Check sheet for the modelled part. Datum: model origin and axes. Units: mm. Face numbers are marked on the shaded views. A direction names the side the tool comes from. Round coordinates to 2 decimals unless told otherwise and drop trailing zeros. Loops run counter-clockwise (first coordinate to the right, second up) from the corner with the lowest first, then second, coordinate; pieces in that order, holes last. Notation, with made-up numbers: (62, 61.25) - (76, 61.25) arc R19 cw to (76, 96.25) - close; hole circle Ø3 at (88, 75). An arc over 180 degrees is marked (long way). Return JSON: item names as keys, results as strings.
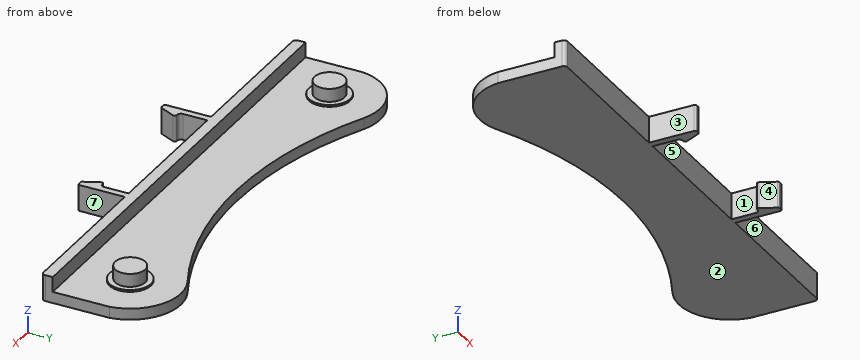
from build123d import *

# Parameters (mm, degrees)
F0_R     = 5.500353
F1_DEPTH = 3
F0_R_2   = 4.000323
F2_DEPTH = 3.5
F3_DEPTH = 7
F4_R     = 1
F5_R     = 0.5


with BuildPart() as f1:
    # F0 (on Top) → F1 (new body)
    with BuildSketch(Plane.XY):
        with BuildLine():
            ThreePointArc((0.003197, 9.6562), (-22.731522, 12.261138), (-44.2788, 19.966198))
            ThreePointArc((-44.2788, 19.966198), (-56.566858, 19.530956), (-63.405201, 9.312206))
            Line((-63.405201, 9.312206), (-63.405201, -5.757801))
            Line((-63.405201, -5.757801), (0.000519, -5.757801))
            Line((0.000519, -5.757801), (0.003197, 9.6562))
        make_face()
        with Locations((-49.99641, 7.740587)):
            Circle(F0_R, mode=Mode.SUBTRACT)
    extrude(amount=F1_DEPTH)

    # F0 (on Top) → F2 (join)
    with BuildSketch(Plane.XY):
        with Locations((-49.99641, 7.740587)):
            Circle(F0_R)
        with Locations((-49.997022, 7.740204)):
            Circle(F0_R_2, mode=Mode.SUBTRACT)
    extrude(amount=F2_DEPTH)

    # F0 (on Top) → F3 (join)
    with BuildSketch(Plane.XY):
        Polygon((-19.75, -8.743801), (-21.641288, -8.743801), (-21.641288, -21.243801), (-20.041288, -21.243801), (-17.75, -16.243801), (-19.75, -16.243801), align=None)
        with Locations((-49.997022, 7.740204)):
            Circle(F0_R_2)
        Polygon((0.000519, -5.757801), (-63.405201, -5.757801), (-63.405201, -8.743801), (-21.641288, -8.743801), (-19.75, -8.743801), (0, -8.743801), align=None)
    extrude(amount=F3_DEPTH)

    # F4
    f4_edges = [f1.edges().sort_by_distance(p)[0] for p in [
        (-19.75, -16.243801, 3.5),
        (-63.405201, -8.743801, 3.5),
    ]]
    fillet(f4_edges, radius=F4_R)

    # F5
    f5_edges = [f1.edges().sort_by_distance(p)[0] for p in [
        (-17.75, -16.243801, 3.5),
        (-20.041288, -21.243801, 3.5),
        (-21.641288, -21.243801, 3.5),
    ]]
    fillet(f5_edges, radius=F5_R)

    # F6: F1 across plane


with BuildPart() as f1_1:
    add(f1.part)
    add(f1.part.mirror(Plane.YZ))


solid = f1_1.part
Q1. Draft check along X on the marked faces 4, 5, 6 and 7. Enter one of: released by +X, released by -X, zero draft, split by the parting line, or undercut.
Answer key:
{"face 4": "undercut", "face 5": "undercut", "face 6": "zero draft", "face 7": "released by +X"}
Q2. Sectioned sample at D-D (x = -10.5). Enter the section's corners in (y, z), plus the area to 3 significant figures.
Answer key:
{"outline": "(-8.74, 0) - (10.2, 0) - (10.2, 3) - (-5.76, 3) - (-5.76, 7) - (-8.74, 7) - close", "area": "68.8 mm²"}
Q3. Sectioned sample at C-C (y = 16). Enter the section's corners in (x, z).
Answer key:
{"outline": "(-60.67, 0) - (-35.11, 0) - (-35.11, 3) - (-60.67, 3) - close; (35.11, 0) - (60.67, 0) - (60.67, 3) - (35.11, 3) - close"}
Q4. Tool access check on the marked faces 1, 2 and 3. Record the directions out of +Z, -Z, +X, -X, +Y, -Y that give a thin tool (end or side, any length) a straight path to the whole face; none if there is none.
Answer key:
{"face 1": "+Z, -Z", "face 2": "-Z, +X, -X, +Y, -Y", "face 3": "+Z, -Z, -X, -Y"}
Q5. Scan lines: probe 1 along X at (y, z) = (7.5, 6); probe 2 along X at (y, z) = (-15, 2.25); probe 3 along Y at (x, z) = (-33, 3.25). Record each from-to range of solid material in increasing order. Write a range as [from, to].
Answer key:
{"probe 1": "x = [-53.99, -46], [46, 53.99]", "probe 2": "x = [-21.64, -19.75], [19.75, 21.64]", "probe 3": "y = [-8.74, -5.76]"}
Q6. Sectioned sample at A-A (y = -13.5). Enter the section's corners in (x, z).
Answer key:
{"outline": "(-21.64, 0) - (-19.75, 0) - (-19.75, 7) - (-21.64, 7) - close; (19.75, 0) - (21.64, 0) - (21.64, 7) - (19.75, 7) - close"}
Q7. Sectioned sample at B-B (z = 5). Enter the section's corners in (x, y), plus the area to 3 significant figures.
Answer key:
{"outline": "(-63.41, -7.74) arc R1 ccw to (-62.41, -8.74) - (-21.64, -8.74) - (-21.64, -20.74) arc R0.5 ccw to (-21.14, -21.24) - (-20.36, -21.24) arc R0.5 ccw to (-19.91, -20.95) - (-18.07, -16.95) arc R0.5 ccw to (-18.53, -16.24) - (-18.75, -16.24) arc R1 cw to (-19.75, -15.24) - (-19.75, -8.74) - (19.75, -8.74) - (19.75, -15.24) arc R1 cw to (18.75, -16.24) - (18.53, -16.24) arc R0.5 ccw to (18.07, -16.95) - (19.91, -20.95) arc R0.5 ccw to (20.36, -21.24) - (21.14, -21.24) arc R0.5 ccw to (21.64, -20.74) - (21.64, -8.74) - (62.41, -8.74) arc R1 ccw to (63.41, -7.74) - (63.41, -5.76) - (-63.41, -5.76) - close; circle Ø8 at (-50, 7.74); circle Ø8 at (50, 7.74)", "area": "535 mm²"}
Q8. Depth check by flat-ended pin: P1, Ø1, axis at x = -22, y = 4.5, coming from the -Z side; P2, Ø1.2, axis at x = 9, z = 4, coming from the +Y side; P3, Ø21.5, axis at x = 6.5, y = 14, coming from the +Z side; P4, Ø1, axis at y = 10.5, z = 2, coming from the +X side. Enter the tip coordinate at first touch or a pass-through.
Answer key:
{"P1": "stops at z = 0", "P2": "stops at y = -5.76", "P3": "stops at z = 3", "P4": "stops at x = 63.31"}
